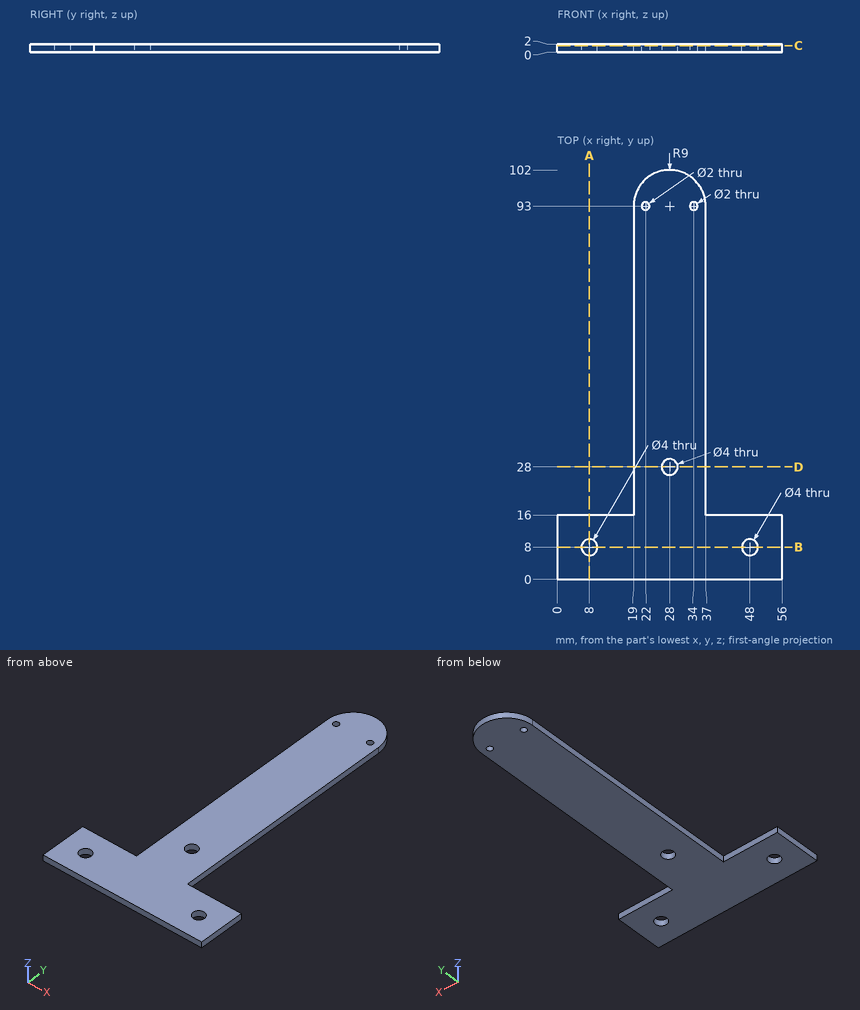
The drawing under review shows one solid part. Ordinate dimensions are in mm from its lowest x, y, z. Coordinates: 2 decimals unless noted, no trailing zeros. Order: outer loops, then holes, each group sorted by start corner. A loop starts at its lowest first (then second) coordinate and runs counter-clockwise, first axis right, second up. Notation, with made-up numbers: (10, -26.75) -> (43, -26.75) arc R15 cw to (43, -0.75) -> close; hole circle Ø10 at (-27, -34.75). An arc over 180 degrees is marked (long way). Return JSON: item names as keys, results as strings.
1. We need section A-A on x = 8. Write out the cut boundary in (y, z), and give its area (3 significant figures).
Answer block:
{"outline": "(0, 0) -> (6, 0) -> (6, 2) -> (0, 2) -> close; (10, 0) -> (16, 0) -> (16, 2) -> (10, 2) -> close", "area": "24.0 mm²"}
2. For pin 1 Ø1 at (x, z) = (46, 1) entering from +Y; pin 2 Ø5 at (x, y) = (48, 8) entering from +Z; pin 3 Ø1.6 at (x, y) = (22, 93) entering from -Z, all flat-tipped, find the tip position at first contact; note any pin that passes through.
Answer block:
{"pin 1": "y = 16", "pin 2": "z = 2", "pin 3": "through"}
3. For line 1 (X direction, y = 93, z = 0.7); line 2 (Y direction, x = 28, z = 0.6); line 3 (Y direction, x = 40.5, z = 1.65), list the stretches that pass through material, from the lowest coordinate up. Write a range as from..to.
Answer block:
{"line 1": "19..21, 23..33, 35..37", "line 2": "0..26, 30..102", "line 3": "0..16"}
4. We need section C-C on z = 1.6. Write out the cut boundary in (x, y), and give its area (3 significant figures).
Answer block:
{"outline": "(0, 0) -> (56, 0) -> (56, 16) -> (37, 16) -> (37, 93) arc R9 ccw to (19, 93) -> (19, 16) -> (0, 16) -> close; hole circle Ø4 at (8, 8); hole circle Ø2 at (22, 93); hole circle Ø4 at (28, 28); hole circle Ø2 at (34, 93); hole circle Ø4 at (48, 8)", "area": "2,370 mm²"}
5. We need section D-D on y = 28. Write out the cut boundary in (x, z).
Answer block:
{"outline": "(19, 0) -> (26, 0) -> (26, 2) -> (19, 2) -> close; (30, 0) -> (37, 0) -> (37, 2) -> (30, 2) -> close"}
6. We need section B-B on y = 8. Write out the cut boundary in (x, z), and give its area (3 significant figures).
Answer block:
{"outline": "(0, 0) -> (6, 0) -> (6, 2) -> (0, 2) -> close; (10, 0) -> (46, 0) -> (46, 2) -> (10, 2) -> close; (50, 0) -> (56, 0) -> (56, 2) -> (50, 2) -> close", "area": "96.0 mm²"}
